```python
from build123d import *

# Parameters (mm, degrees)
F0_W           = 206.375
F0_H           = 36.5125
F1_DEPTH       = 4.7625
F5_D           = 2.2606
F5_DEPTH       = 14.61135
F5_TIP         = 0.6791527577
F5_ON_F3_D     = 2.2606
F5_ON_F3_DEPTH = 14.61135
F5_ON_F3_TIP   = 0.6791527577
F5_ON_F2_D     = 2.2606
F5_ON_F2_DEPTH = 14.61135
F5_ON_F2_TIP   = 0.6791527577
F7_DEPTH       = 25.4


with BuildPart() as f1:
    # F0 (on Right) → F1 (new body)
    with BuildSketch(Plane.YZ):
        Rectangle(F0_W, F0_H)
    extrude(amount=F1_DEPTH)

    # F5
    with Locations(Plane.XY.offset(18.25625)):
        with Locations((2.38125, -77.7875), (2.38125, 77.7875)):
            Hole(F5_D / 2, depth=F5_DEPTH)
            with Locations((0, 0, -(F5_DEPTH + F5_TIP / 2))):  # 118° drill point
                Cone(0, F5_D / 2, F5_TIP, mode=Mode.SUBTRACT)

    # F5 on F3
    with Locations(Plane.XZ.offset(103.1875)):
        with Locations((2.38125, -5.55625)):
            Hole(F5_ON_F3_D / 2, depth=F5_ON_F3_DEPTH)
            with Locations((0, 0, -(F5_ON_F3_DEPTH + F5_ON_F3_TIP / 2))):  # 118° drill point
                Cone(0, F5_ON_F3_D / 2, F5_ON_F3_TIP, mode=Mode.SUBTRACT)

    # F5 on F2
    with Locations(Plane(origin=(0, 103.1875, 0), x_dir=(-1, 0, 0), z_dir=(0, 1, 0))):
        with Locations((-2.38125, -5.55625)):
            Hole(F5_ON_F2_D / 2, depth=F5_ON_F2_DEPTH)
            with Locations((0, 0, -(F5_ON_F2_DEPTH + F5_ON_F2_TIP / 2))):  # 118° drill point
                Cone(0, F5_ON_F2_D / 2, F5_ON_F2_TIP, mode=Mode.SUBTRACT)

    # F6 (on face) → F7 (cut)
    with BuildSketch(Plane.YZ.offset(4.7625)):
        with BuildLine():
            Line((-65.5934088888, 6.985), (-86.8065911112, 6.985))
            ThreePointArc((-86.8065911112, 6.985), (-88.9, 0), (-86.8065911112, -6.985))
            Line((-86.8065911112, -6.985), (-65.5934088888, -6.985))
            ThreePointArc((-65.5934088888, -6.985), (-63.5, 0), (-65.5934088888, 6.985))
        make_face()
        with BuildLine():
            ThreePointArc((10.6065911112, -6.985), (12.7, 0), (10.6065911112, 6.985))
            Line((10.6065911112, 6.985), (-10.6065911112, 6.985))
            ThreePointArc((-10.6065911112, 6.985), (-12.7, 0), (-10.6065911112, -6.985))
            Line((-10.6065911112, -6.985), (10.6065911112, -6.985))
        make_face()
    extrude(amount=-F7_DEPTH, mode=Mode.SUBTRACT)


solid = f1.part
```
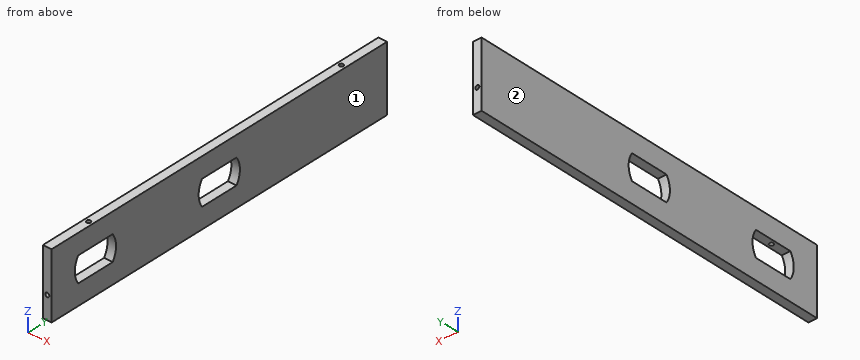
Input: part model. Units: mm. Frame: model coordinates. Face numbers are marked on the shaded views. Round coordinates to 2 decimals unless told otherwise and drop trailing zeros. Loops run counter-clockwise (first coordinate to the right, second up) from the corner with the lowest first, then second, coordinate; pieces in that order, holes last. Notation, with made-up numbers: (58, 45) -> (83, 45) arc R19 cw to (83, 51) -> close; hole circle Ø7 at (-13.75, 86). An arc over 180 degrees is marked (long way). Use one line per item in the form item = value. Start each with the question number.
Item 1: Contact query for a flat-ended pin moving along its axis: pin 1 Ø1.4 at (x, z) = (2.38, -5.56) entering from +Y. Output: stop coordinate, or through.
Item 2: Section query A-A on y = 2. Return the cut outline in (x, z) (1 decimal), then the cut area to 3 significant figures.
Item 3: Mould query, pull axis X, two halves, no side actions, for the marked faces 1 and 2. Classes: pulls with the +X half, pulls with the -X half, needs draft (parallel to the pull), parting line crosses it, or undercut.
Item 4: Material intervals for L1, parallel to Z at x = 1.9, y = -67.5 (3 decimals); L2, parallel to Y at x = 3.7, z = -5.5; L3, parallel to Y at x = 1.4, z = 8.5, sorted ascending. Write a range as from..to.
Ans:
q1.pin_1 = 88.32
q2.outline = (0, -18.3) -> (4.8, -18.3) -> (4.8, -7) -> (0, -7) -> close; (0, 7) -> (4.8, 7) -> (4.8, 18.3) -> (0, 18.3) -> close
q2.area = 107 mm^2
q3.face_1 = pulls with the +X half
q3.face_2 = pulls with the -X half
q4.L1 = -18.256..-6.985, 6.985..18.256
q4.L2 = -103.19..-87.65, -64.75..-11.45, 11.45..103.19
q4.L3 = -103.19..-78.35, -77.23..77.23, 78.35..103.19
